```python
from build123d import *

# Parameters (mm, degrees)
BOSS_EXTRUDE1_DEPTH     = 4
MOVE_FACE4_BY           = 2.5
CIRPATTERN1_COUNT       = 6
CUT_EXTRUDE1_DEPTH      = 70.81610106
CUT_EXTRUDE1_DEPTH_BACK = 66.81610106
CUT_EXTRUDE1_START      = -4
SKETCH9_R               = 5
M4_CLEARANCE_HOLE1_D    = 4.5
CUT_EXTRUDE3_DEPTH      = 66.81610106
CUT_EXTRUDE3_DEPTH_BACK = 66.81610106
SKETCH11_R              = 18.5
CUT_EXTRUDE4_DEPTH      = 66.81610106
MOVE_FACE3_BY           = 0.1
MOVE_FACE3_2_BY         = 0.1
FILLET1_R               = 1
MOVE_FACE1_BY           = 0.1
MOVE_FACE1_2_BY         = 0.1


with BuildPart() as part:
    # Sketch2 → Boss-Extrude1 (new body)
    with BuildSketch(Plane.YZ):
        with BuildLine():
            Line((-12.727922061, -32.852837258), (-17.616293225, -27.964466094))
            ThreePointArc((-17.616293225, -27.964466094), (-19.238409969, -26.880602337), (-21.151827131, -26.5))
            Line((-21.151827131, -26.5), (-27, -26.5))
            ThreePointArc((-27, -26.5), (-53.5, 0), (-27, 26.5))
            Line((-27, 26.5), (0, 26.5))
            Line((0, 26.5), (0, -38.124915197))
            ThreePointArc((0, -38.124915197), (-6.888301783, -36.754746782), (-12.727922061, -32.852837258))
        make_face()
    extrude(amount=-BOSS_EXTRUDE1_DEPTH)

    # Move Face4: a face moved outward by 2.5
    extrude(part.faces().sort_by_distance((0, -23.32621052, -1.71865324))[0], amount=MOVE_FACE4_BY, dir=(1, 0, 0))

    # Sketch18 → CSK for M2.5 Flat Head Machine Screw1 (revolve, cut)
    with BuildSketch(Plane(origin=(2.5, -46.485571585, 11.25), x_dir=(0, 0, -1), z_dir=(0, 1, 0))):
        Polygon((0, 0), (0, 6.5), (1.45, 6.5), (1.45, 4.3), (2.75, 3), (2.75, 0), align=None)
    csk_for_m2_5_flat_head_machine_screw1 = revolve(axis=Axis((8.85, -46.485571585, 11.25), (-1, 0, 0)), mode=Mode.SUBTRACT)

    # CirPattern1: CSK for M2.5 Flat Head Machine Screw1 ×6 about axis, 1 skipped
    cirpattern1_axis = Axis((0, -27, 0), (1, 0, 0))
    add([csk_for_m2_5_flat_head_machine_screw1.rotate(cirpattern1_axis, i * 360 / CIRPATTERN1_COUNT) for i in range(1, CIRPATTERN1_COUNT) if i not in (5,)], mode=Mode.SUBTRACT)

    # Sketch9 → Cut-Extrude1 (cut, two sides: drawn at the far end of the back side and taken through both)
    with BuildSketch(Plane.YZ.offset(CUT_EXTRUDE1_START - CUT_EXTRUDE1_DEPTH_BACK)):
        with Locations((0, 3.875084803)):
            Circle(SKETCH9_R)
        with Locations((0, -20.124915197)):
            Circle(SKETCH9_R)
    extrude(amount=CUT_EXTRUDE1_DEPTH + CUT_EXTRUDE1_DEPTH_BACK, mode=Mode.SUBTRACT)

    # M4 Clearance Hole1 (through all)
    with Locations(Plane.ZY.offset(4)):
        with Locations((15.875084803, 0), (-28.610196571, -8.485281374), (-32.124915197, 0)):
            Hole(M4_CLEARANCE_HOLE1_D / 2)

    # Sketch11 → Cut-Extrude3 (cut, two sides: drawn at the far end of the back side and taken through both)
    with BuildSketch(Plane.YZ.offset(-CUT_EXTRUDE3_DEPTH_BACK)):
        with Locations(Location((-27, 0, 0), (0, 0, 270))):
            Circle(SKETCH11_R)
    extrude(amount=CUT_EXTRUDE3_DEPTH + CUT_EXTRUDE3_DEPTH_BACK, mode=Mode.SUBTRACT)

    # Sketch14 → Cut-Extrude4 (cut, through all)
    with BuildSketch(Plane.YZ):
        with BuildLine():
            Line((16, 3.875084803), (16, -92.124915197))
            ThreePointArc((16, -92.124915197), (0, -108.124915197), (-16, -92.124915197))
            Line((-16, -92.124915197), (-16, 3.875084803))
            ThreePointArc((-16, 3.875084803), (0, 19.875084803), (16, 3.875084803))
        make_face()
    extrude(amount=CUT_EXTRUDE4_DEPTH, mode=Mode.SUBTRACT)

    # Move Face3: a face moved inward by 0.1
    extrude(part.faces().sort_by_distance((1.25, -16, -22.22761705))[0], amount=MOVE_FACE3_BY, dir=(0, -1, 0), mode=Mode.SUBTRACT)

    # Move Face3 2: a curved face moved inward by 0.1
    add(Solid.thicken(part.faces().sort_by_distance((1.25, -7.643007581, 17.931557871))[0], -MOVE_FACE3_2_BY), mode=Mode.SUBTRACT)

    # Fillet1
    # the kernel refuses this fillet: 1 mm, written as the material it takes off along each edge
    with BuildSketch(Plane(origin=(8.514983565, -16.1, -29.480759319), x_dir=(0, -0.7085538921245894, 0.7056567026218171), z_dir=(-1, 0, 0))) as fillet1_piece_1:
        with BuildLine():
            CenterArc((2.40635928, 0.999119304), FILLET1_R, 135.117377496, 132.477802543)
            Line((1.697805388, 1.704776006), (1.626949998, 1.775341677))
            Line((1.626949998, 1.775341677), (-0.070855389, 0.07056567))
            Line((-0.070855389, 0.07056567), (0.000204862, -0.09999979))
            ThreePointArc((0.000204862, -0.09999979), (2.144562806, -0.095606801), (2.360203605, -0.09991193))
            Line((2.360203605, -0.09991193), (2.364399576, 0))
        make_face()
    extrude(amount=8.514983565, mode=Mode.SUBTRACT)
    with BuildSketch(Plane(origin=(7.130226118, -16.1, -14.947909553), x_dir=(3.712378047995727e-15, -0.8357607449815292, -0.5490937780998063), z_dir=(-1, 0, 0))) as fillet1_piece_2:
        with BuildLine():
            CenterArc((1.852732086, -0.998810714), FILLET1_R, 92.794627145, 120.510237406)
            Line((1.016971341, -1.547904492), (0, 0))
            ThreePointArc((0, 0), (0.901987989, -0.022001795), (1.803975978, 0))
        make_face()
    extrude(amount=7.130226118, mode=Mode.SUBTRACT)
    with BuildSketch(Plane(origin=(5.398868608, -13.499485451, 12.648561456), x_dir=(-5.5330585224254415e-15, 0.5746651545031678, 0.8183886364068421), z_dir=(-1, 0, 0))) as fillet1_piece_3:
        with BuildLine():
            CenterArc((1.191014528, -0.999356323), FILLET1_R, 92.055865996, 96.142233036)
            ThreePointArc((0.201233565, -1.141952418), (0.109565926, -0.569399201), (0, 0))
            ThreePointArc((0, 0), (0.577570298, -0.010363194), (1.155140596, 0))
        make_face()
    extrude(amount=5.398868608, mode=Mode.SUBTRACT)

    # Move Face1: a face moved inward by 0.1
    extrude(part.faces().sort_by_distance((-4, -26.75, 20.03750848))[0], amount=MOVE_FACE1_BY, dir=(1, 0, 0), mode=Mode.SUBTRACT)

    # Move Face1 2: a face moved inward by 0.1
    extrude(part.faces().sort_by_distance((2.5, -26.75, 21.042523411))[0], amount=MOVE_FACE1_2_BY, dir=(-1, 0, 0), mode=Mode.SUBTRACT)

    # Mirror1: part across plane


with BuildPart() as part_1:
    add(part.part)
    add(part.part.mirror(Plane(origin=(0, 0, 0), x_dir=(0, 0, 1), z_dir=(0, -1, 0))))


solid = part_1.part
```
Part model, mm, in its own coordinate system. A direction names the side the tool comes from. Round coordinates to 2 decimals unless told otherwise and drop trailing zeros. Loops run counter-clockwise (first coordinate to the right, second up) from the corner with the lowest first, then second, coordinate; pieces in that order, holes last. Notation, with made-up numbers: (26.25, 56) -> (54.25, 56) arc R17 ccw to (54.25, 65) -> close; hole circle Ø5 at (42.25, 38.25). An arc over 180 degrees is marked (long way). Use one line per item in the form item = value. Start each with the question number.
Item 1: Band-saw the part on D-D (z = 15.5). List the corners of the cut face in (x, y), plus the area to 3 significant figures.
Item 2: Tool access for faces 4 (the cylindrical face through (-0.79, 45.06, 4.01)), 5 (the cylindrical face through (-0.246, -9.954, -9.981)): list every direction of +Z, -Z, +X, -X, +Y, -Y with a clear straight run to the whole face (end or side of a thin tool).
Item 3: Band-saw the part on A-A (z = 4). List the corners of the cut face in (x, y).
Item 4: Drill centre lines: line 1 along Z through (x, y) = (-2.25, 3); line 2 along Y through (x, z) = (-0.75, -20.5); line 3 along Y through (x, z) = (-0.5, -20.5). Where is each one in solid material? Low to high.
Item 5: Drop flat-ended pins along their axis: pin 1 Ø3.5 at (y, z) = (-46.49, -11.25) entering from +X; pin 2 Ø2 at (x, z) = (-1, -12) entering from +Y; pin 3 Ø3 at (x, z) = (0.5, 10.5) entering from -Y. Give the stop position or say it passes through.
Item 6: Two-plate mould, pull along Z, no slides. Class faces 1 (the cylindrical face through (0.97, -25.95, -25.04)), 2 (the flat face through (-1, 24, -26.5)), 3 (the cylindrical face through (-0.794, -53.494, -0.583)): released by +Z, released by -Z, zero draft, split by the parting line, or undercut.
Item 7: Band-saw the part on B-B (y = 36). List the corners of the cut face in (x, z).
Item 8: Band-saw the part on C-C (z = -3.5). List the corners of the cut face in (x, y).
Data:
q1.outline = (-3.9, -48.49) -> (2.4, -48.49) -> (2.4, -37.1) -> (-3.9, -37.1) -> close; (-3.9, -16.9) -> (2.4, -16.9) -> (2.4, -11.14) -> (0, -11.14) -> (0, -2.22) -> (-3.9, -2.22) -> close; (-3.9, 2.22) -> (0, 2.22) -> (0, 11.14) -> (2.4, 11.14) -> (2.4, 16.9) -> (-3.9, 16.9) -> close; (-3.9, 37.1) -> (2.4, 37.1) -> (2.4, 48.49) -> (-3.9, 48.49) -> close
q1.area = 286 mm^2
q2.face_4 = +X, -X
q2.face_5 = +X
q3.outline = (-3.9, -53.2) -> (2.4, -53.2) -> (2.4, -45.06) -> (-3.9, -45.06) -> close; (-3.9, -8.94) -> (0, -8.94) -> (0, -5) -> (-3.9, -5) -> close; (-3.9, 5) -> (0, 5) -> (0, 8.94) -> (-3.9, 8.94) -> close; (-3.9, 45.06) -> (2.4, 45.06) -> (2.4, 53.2) -> (-3.9, 53.2) -> close
q4.line_1 = -37.87 to -24.12, -16.12 to -0.12, 7.88 to 26.5
q4.line_2 = -43.79 to -28.5, -25.5 to -4.99, 4.99 to 25.5, 28.5 to 43.79
q4.line_3 = -43.79 to -28.89, -25.11 to -4.99, 4.99 to 25.11, 28.89 to 43.79
q5.pin_1 = -1.5
q5.pin_2 = 51.11
q5.pin_3 = -51.92
q6.face_1 = undercut
q6.face_2 = released by -Z
q6.face_3 = split by the parting line
q7.outline = (-3.9, -24.92) -> (2.4, -24.92) -> (2.4, -16.16) -> (-3.9, -16.16) -> close; (-3.9, 16.16) -> (2.4, 16.16) -> (2.4, 24.92) -> (-3.9, 24.92) -> close
q8.outline = (-3.9, -53.27) -> (2.4, -53.27) -> (2.4, -45.17) -> (-3.9, -45.17) -> close; (-3.9, -8.83) -> (0, -8.83) -> (0, 8.83) -> (-3.9, 8.83) -> close; (-3.9, 45.17) -> (2.4, 45.17) -> (2.4, 53.27) -> (-3.9, 53.27) -> close
